```python
from build123d import *

# Parameters (mm, degrees)
F0_W     = 1000
F0_H     = 900
F1_DEPTH = 50
F3_DEPTH = 1016
F5_DEPTH = 908


with BuildPart() as f1:
    # F0 (on Front) → F1 (new body)
    with BuildSketch(Plane.XZ):
        Rectangle(F0_W, F0_H)
    extrude(amount=F1_DEPTH)

    # F2 (on face) → F3 (cut)
    with BuildSketch(Plane(origin=(-500, 0, 0), x_dir=(0, -1, 0), z_dir=(-1, 0, 0))):
        Polygon((50, -332.5), (50, -317.5), (40, -317.5), (40, -312.5), (30, -312.5), (30, -337.5), (40, -337.5), (40, -332.5), align=None)
        Polygon((40, -92.5), (50, -92.5), (50, -77.5), (40, -77.5), (40, -72.5), (30, -72.5), (30, -97.5), (40, -97.5), align=None)
        Polygon((40, 127.5), (50, 127.5), (50, 142.5), (40, 142.5), (40, 147.5), (30, 147.5), (30, 122.5), (40, 122.5), align=None)
        Polygon((40, 367.5), (50, 367.5), (50, 382.5), (40, 382.5), (40, 387.5), (30, 387.5), (30, 362.5), (40, 362.5), align=None)
    extrude(amount=-F3_DEPTH, mode=Mode.SUBTRACT)

    # F4 (on face) → F5 (cut)
    with BuildSketch(Plane.XY.offset(450)):
        Polygon((292.5, -50), (307.5, -50), (307.5, -40), (312.5, -40), (312.5, -30), (287.5, -30), (287.5, -40), (292.5, -40), align=None)
        Polygon((92.5, -40), (92.5, -50), (107.5, -50), (107.5, -40), (112.5, -40), (112.5, -30), (87.5, -30), (87.5, -40), align=None)
        Polygon((-107.5, -40), (-107.5, -50), (-92.5, -50), (-92.5, -40), (-87.5, -40), (-87.5, -30), (-112.5, -30), (-112.5, -40), align=None)
        Polygon((-307.5, -40), (-307.5, -50), (-292.5, -50), (-292.5, -40), (-287.5, -40), (-287.5, -30), (-312.5, -30), (-312.5, -40), align=None)
    extrude(amount=-F5_DEPTH, mode=Mode.SUBTRACT)


solid = f1.part
```
The model under review builds one solid part; all positions refer to its coordinate system, in mm. A direction names the side the tool comes from. Round coordinates to 2 decimals unless told otherwise and drop trailing zeros.
1) The part is to be moulded in two halves that separate along Y. For faces 3 (the face through (311, -40, 254)), 4 (the face through (200, -40, 386)), 5 (the face through (199, -50, 26)), 6 (the face through (500, -25, -6)), say which applies: pulls with the +Y half, pulls with the -Y half, needs draft (parallel to the pull), parting line crosses it, or undercut.
Values follow:
face 3: undercut
face 4: undercut
face 5: pulls with the -Y half
face 6: needs draft
2) Clearance check with a flat-ended pin moving along its axis: P1, Ø12, axis at x = -312.5, z = 77.5, coming from the +Y side. State where the tip first meets the part, or that it passes through.
Values follow:
P1: stops at y = 0
3) Wall thickness on line 1 along Z through (x, y) = (139, -35.5); line 2 along Z through (x, y) = (55, -46.5); line 3 along X through (y, z) = (-34.5, 296.5): over which ranges is each line inside the solid? List them lowest first.
Values follow:
line 1: z = -450 to -337.5, -312.5 to -97.5, -72.5 to 122.5, 147.5 to 362.5, 387.5 to 450
line 2: z = -450 to -332.5, -317.5 to -92.5, -77.5 to 127.5, 142.5 to 367.5, 382.5 to 450
line 3: x = -500 to -312.5, -287.5 to -112.5, -87.5 to 87.5, 112.5 to 287.5, 312.5 to 500
4) Tool access review of faces 1 (the face through (-200, -40, 386)), 2 (the face through (-1, -50, -203)): name each direction out of +Z, -Z, +X, -X, +Y, -Y from which nothing blocks a thin tool from reaching the whole face with its end or side.
Values follow:
face 1: none
face 2: +Z, -Z, +X, -X, -Y
